Build history of the part. All positions in model axes, mm. Give positions to 0.01 mm unless a question says otherwise; leave off trailing zeros. Write each loop counter-clockwise with the first axis right and the second up, starting at its lowest first coordinate (ties: lowest second). Pieces come first, ordered by that corner, then holes. Notation, with made-up numbers: (75, 48.5) -> (128, 48.5) arc R15 cw to (128, 74.5) -> close; hole circle Ø1 at (51, -23.5). An arc over 180 degrees is marked (long way). Put each result on its own line as item: value.
from build123d import *

# Parameters (mm, degrees)
BOSS_EXTRUDE1_DEPTH      = 1.5875
A_0_234_DIAMETER_HOLE1_D = 5.9436


with BuildPart() as part:
    # Sketch1 → Boss-Extrude1 (new body)
    with BuildSketch(Plane(origin=(0, 0, 0), x_dir=(0, 0, -1), z_dir=(1, 0, 0))):
        with BuildLine():
            Line((438.6326, 491.49), (491.49, 491.49))
            ThreePointArc((491.49, 491.49), (495.980128061, 489.630128061), (497.84, 485.14))
            Line((497.84, 485.14), (497.84, 6.35))
            ThreePointArc((497.84, 6.35), (495.980128061, 1.859871939), (491.49, 0))
            Line((491.49, 0), (6.35, 0))
            ThreePointArc((6.35, 0), (1.859871939, 1.859871939), (0, 6.35))
            Line((0, 6.35), (0, 485.14))
            ThreePointArc((0, 485.14), (1.859871939, 489.630128061), (6.35, 491.49))
            Line((6.35, 491.49), (59.2074, 491.49))
            ThreePointArc((59.2074, 491.49), (63.697528061, 489.630128061), (65.5574, 485.14))
            Line((65.5574, 485.14), (65.5574, 481.965))
            ThreePointArc((65.5574, 481.965), (67.417271939, 477.474871939), (71.9074, 475.615))
            Line((71.9074, 475.615), (425.9326, 475.615))
            ThreePointArc((425.9326, 475.615), (430.422728061, 477.474871939), (432.2826, 481.965))
            Line((432.2826, 481.965), (432.2826, 485.14))
            ThreePointArc((432.2826, 485.14), (434.142471939, 489.630128061), (438.6326, 491.49))
        make_face()
    extrude(amount=-BOSS_EXTRUDE1_DEPTH)

    # A (0.234) Diameter Hole1 (through all)
    with Locations(Plane(origin=(1.02362, -1353.361752646, -2205.813131805), x_dir=(0, 0, -1), z_dir=(1, 0, 0))):
        with Locations((-2173.593231805, 1361.299252646), (-1740.193031805, 1361.29924771), (-1765.593031805, 1836.91424771), (-2148.193231805, 1836.91424771)):
            Hole(A_0_234_DIAMETER_HOLE1_D / 2)


solid = part.part
1) Wall check: L1, parallel to Y at x = -0.35, z = -172 (3 decimals); L2, parallel to Y at x = -1.3, z = -69.5. Give the ranges that are in metal, low to high.
Filled sheet:
L1: 0 to 475.615
L2: 0 to 476.09
2) Slice it at B-B (z = -269.5). Write the cut outline in (x, y) (1 decimal), plus the area to 3 significant figures.
Filled sheet:
outline: (-1.6, 0) -> (0, 0) -> (0, 475.6) -> (-1.6, 475.6) -> close
area: 755 mm2
3) Slice it at A-A (x = -1.2). Give the number of separate pieces and of enclosed holes in the cut face, plus the area to 3 significant figures.
Filled sheet:
separate pieces: 1
enclosed holes: 4
area: 239,000 mm2
4) Pin check, flat tip, straight feed: pin 1 (0.5 mm diameter, centred on x = -1, z = -185, fed in from +Y) (3 decimals). Stop position of the tip, or through.
Filled sheet:
pin 1: y = 475.615
